from build123d import *

# Parameters (mm, degrees)
F0_W     = 558.8
F0_H     = 330.2
F0_W_2   = 527.05
F0_H_2   = 298.45
F1_DEPTH = 25.4
F2_DEPTH = 19.05
F3_W     = 406.4
F3_H     = 209.55
F4_DEPTH = 19.05


with BuildPart() as f1:
    # F0 (on Front) → F1 (new body)
    with BuildSketch(Plane.XZ):
        with Locations((-9.705722, 22.848336)):
            Rectangle(F0_W, F0_H)
        with Locations((-9.705722, 22.848336)):
            Rectangle(F0_W_2, F0_H_2, mode=Mode.SUBTRACT)
    extrude(amount=F1_DEPTH)

    # F0 (on Front) → F2 (join)
    with BuildSketch(Plane.XZ):
        with Locations((-9.705722, 22.848336)):
            Rectangle(F0_W_2, F0_H_2)
    extrude(amount=F2_DEPTH)

    # F3 (on face) → F4 (join)
    with BuildSketch(Plane.XZ):
        with Locations((-9.705722, 26.023336)):
            Rectangle(F3_W, F3_H)
    extrude(amount=-F4_DEPTH)


solid = f1.part
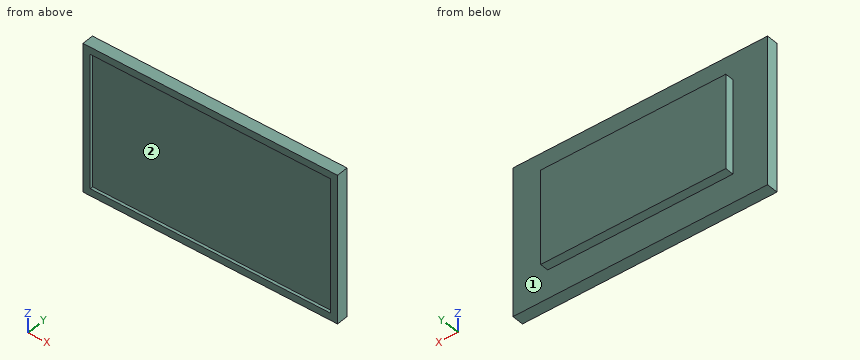
Design review of the part built by this model. Coordinates are the model's own, in mm. Face numbers are marked on the shaded views. Give positions to 0.01 mm unless a question says otherwise; leave off trailing zeros. Loops run counter-clockwise (first coordinate to the right, second up) from the corner with the lowest first, then second, coordinate; pieces in that order, holes last. Notation, with made-up numbers: (-19.5, 47) - (-13.5, 47) arc R33 cw to (-13.5, 80) - close; hole circle Ø3 at (-4.75, 71.5). An arc over 180 degrees is marked (long way). Write item = value, one per line.
1) Draft analysis for pull direction X (two halves, no side actions). For the marked faces 1 and 2, state which applies: +X half, -X half, draft (parallel to the pull), parting line (faces both ways), or undercut.
Result sheet:
face_1 = draft
face_2 = undercut
2) Take a section at B-B on x = -18.5. State the section outline as (y, z) points.
Result sheet:
outline = (-25.4, -142.25) - (0, -142.25) - (0, -78.75) - (19.05, -78.75) - (19.05, 130.8) - (0, 130.8) - (0, 187.95) - (-25.4, 187.95) - (-25.4, 172.07) - (-19.05, 172.07) - (-19.05, -126.38) - (-25.4, -126.38) - close
3) Clearance check with flat-ended pins moving along their axes: pin 1 Ø1 at (x, y) = (173.5, 12.5) entering from +Z; pin 2 Ø5.5 at (x, y) = (-93.5, 9.5) entering from -Z; pin 3 Ø5 at (y, z) = (11.5, 1) entering from -X. State where each tip first meets the part, or that it passes through.
Result sheet:
pin_1 = 130.8
pin_2 = -78.75
pin_3 = -212.91
4) Take a section at C-C on y = 8.5. State the section outline as (x, z) points.
Result sheet:
outline = (-212.91, -78.75) - (193.49, -78.75) - (193.49, 130.8) - (-212.91, 130.8) - close
5) To check wall thickness, follow line 1 (X direction, y = -21.5, z = 140.5); line 2 (Z direction, x = -15, y = -21.5); line 3 (X direction, y = 6.5, z = 66.5). State the ranges of each line that lie inside material, in increasing order.
Result sheet:
line_1 = -289.11 to -273.23, 253.82 to 269.69
line_2 = -142.25 to -126.38, 172.07 to 187.95
line_3 = -212.91 to 193.49
6) Take a section at A-A on z = 108. State the section outline as (x, y) points, and give its area (3 significant figures).
Result sheet:
outline = (-289.11, -25.4) - (-273.23, -25.4) - (-273.23, -19.05) - (253.82, -19.05) - (253.82, -25.4) - (269.69, -25.4) - (269.69, 0) - (193.49, 0) - (193.49, 19.05) - (-212.91, 19.05) - (-212.91, 0) - (-289.11, 0) - close
area = 18,600 mm2
7) Take a section at D-D on z = -111. State the section outline as (x, y) points.
Result sheet:
outline = (-289.11, -25.4) - (-273.23, -25.4) - (-273.23, -19.05) - (253.82, -19.05) - (253.82, -25.4) - (269.69, -25.4) - (269.69, 0) - (-289.11, 0) - close
